from build123d import *

# Parameters (mm, degrees)
F0_R     = 20
F1_DEPTH = 140
F0_R_2   = 25
F2_DEPTH = 10
F3_R     = 25
F4_DEPTH = 10


with BuildPart() as f1:
    # F0 (on Front) → F1 (new body)
    with BuildSketch(Plane.XZ):
        Circle(F0_R)
    extrude(amount=F1_DEPTH)

    # F0 (on Front) → F2 (join)
    with BuildSketch(Plane.XZ):
        Circle(F0_R_2)
        Circle(F0_R, mode=Mode.SUBTRACT)
        Circle(F0_R)
    extrude(amount=-F2_DEPTH)

    # F3 (on face) → F4 (join)
    with BuildSketch(Plane.XZ.offset(140)):
        Circle(F3_R)
    extrude(amount=F4_DEPTH)


solid = f1.part
The model under review builds one solid part; all positions refer to its coordinate system, in mm. A direction names the side the tool comes from. Give positions to 0.01 mm unless a question says otherwise; leave off trailing zeros. Loops run counter-clockwise (first coordinate to the right, second up) from the corner with the lowest first, then second, coordinate; pieces in that order, holes last. Notation, with made-up numbers: (70.5, 66) -> (75.5, 66) arc R24 cw to (75.5, 85) -> close; hole circle Ø10 at (-10, 54). An arc over 180 degrees is marked (long way). Answer as a JSON object with one key per item and string values. Group by question number.
Q1. Tool access review of faces 1 (the flat face through (0, -150, 0)), 2 (the flat face through (-11, 0, 17)): name each direction out of +Z, -Z, +X, -X, +Y, -Y from which nothing blocks a thin tool from reaching the whole face with its end or side.
Q2. Take a section at B-B (x = 0). Write out the cut boundary in (y, z), plus the area to 3 significant figures.
Q3. Draft analysis for pull direction Y (two halves, no side actions). For faces 3 (the flat face through (0, 10, 0)), 4 (the cylindrical face through (23.846, -144.93, 7.509)), 5 (the cylindrical face through (-4.336, -69.02, -19.524)), state which applies: pulls with the +Y half, pulls with the -Y half, needs draft (parallel to the pull), parting line crosses it, or undercut.
Q4. Take a section at A-A (z = 0). Write out the cut boundary in (x, y), plus the area to 3 significant figures.
Q5. Insertion check: pin 1 (3 mm diameter, centred on y = -78.5, z = 4.5, fed in from -X); pin 2 (12 mm diameter, centred on x = 14.5, y = -93, fed in from +Z); pin 3 (1 mm diameter, centred on x = -12, y = -89.5, fed in from -Z). Each pin has a flat end and moves straight along its axis. Give the tip position at first contact, or say it passes through.
Q6. Wall thickness on line 1 along Y through (x, z) = (5, -21); line 2 along X through (y, z) = (-77.5, 18); line 3 along X through (y, z) = (-142, -16): over which ranges is each line inside the solid? List them lowest first.
Q7. Take a section at C-C (y = -110.5). Write out the cut boundary in (x, z).
Answer below:
{
 "1": {"face 1": "+Z, -Z, +X, -X, -Y", "face 2": "none"},
 "2": {"outline": "(-150, -25) -> (-140, -25) -> (-140, -20) -> (0, -20) -> (0, -25) -> (10, -25) -> (10, 25) -> (0, 25) -> (0, 20) -> (-140, 20) -> (-140, 25) -> (-150, 25) -> close", "area": "6,600 mm2"},
 "3": {"face 3": "pulls with the +Y half", "face 4": "needs draft", "face 5": "undercut"},
 "4": {"outline": "(-25, -150) -> (25, -150) -> (25, -140) -> (20, -140) -> (20, 0) -> (25, 0) -> (25, 10) -> (-25, 10) -> (-25, 0) -> (-20, 0) -> (-20, -140) -> (-25, -140) -> close", "area": "6,600 mm2"},
 "5": {"pin 1": "stops at x = -19.77", "pin 2": "stops at z = 18.1", "pin 3": "stops at z = -16.36"},
 "6": {"line 1": "y = -150 to -140, 0 to 10", "line 2": "x = -8.72 to 8.72", "line 3": "x = -19.21 to 19.21"},
 "7": {"outline": "circle Ø40 at (0, 0)"}
}
